from build123d import *

# Parameters (mm, degrees)
EXTRUDE_1_DEPTH     = 0.5
SKETCH_2_R          = 2
SKETCH_2_R_2        = 1.25
EXTRUDE_2_DEPTH     = 5.5
SKETCH_3_R          = 1.25
CUT_EXTRUDE_1_DEPTH = 5.5
SKETCH_4_R          = 4
SKETCH_4_R_2        = 2
CUT_EXTRUDE_2_DEPTH = 5.5


with BuildPart() as part:
    # 草图1 → 凸台-拉伸1 (new body)
    with BuildSketch(Plane.XY):
        with BuildLine():
            Line((0, 2), (3.2, 2))
            ThreePointArc((3.2, 2), (3.765685425, 2.234314575), (4, 2.8))
            Line((4, 2.8), (4, 2.95))
            ThreePointArc((4, 2.95), (3.765685425, 3.515685425), (3.2, 3.75))
            Line((3.2, 3.75), (-3.5, 3.75))
            Line((-3.5, 3.75), (-7, 2))
            Line((-7, 2), (-12.5, 2))
            Line((-12.5, 2), (-12.5, -2))
            Line((-12.5, -2), (-7, -2))
            Line((-7, -2), (-3.5, -3.75))
            Line((-3.5, -3.75), (3.2, -3.75))
            ThreePointArc((3.2, -3.75), (3.765685425, -3.515685425), (4, -2.95))
            Line((4, -2.95), (4, -2.8))
            ThreePointArc((4, -2.8), (3.765685425, -2.234314575), (3.2, -2))
            Line((3.2, -2), (0, -2))
            ThreePointArc((0, -2), (-2, 0), (0, 2))
        make_face()
    extrude(amount=EXTRUDE_1_DEPTH)

    # 草图2 → 凸台-拉伸2 (add)
    with BuildSketch(Plane.ZY.offset(12.5)):
        with Locations((1.5, 0)):
            Circle(SKETCH_2_R)
        with Locations((1.5, 0)):
            Circle(SKETCH_2_R_2, mode=Mode.SUBTRACT)
    extrude(amount=-EXTRUDE_2_DEPTH)

    # 草图3 → 切除-拉伸1 (cut)
    with BuildSketch(Plane.ZY.offset(12.5)):
        with Locations((1.5, 0)):
            Circle(SKETCH_3_R)
    extrude(amount=-CUT_EXTRUDE_1_DEPTH, mode=Mode.SUBTRACT)

    # 草图4 → 切除-拉伸2 (cut)
    with BuildSketch(Plane.ZY.offset(12.5)):
        with Locations((1.5, 0)):
            Circle(SKETCH_4_R)
        with Locations((1.5, 0)):
            Circle(SKETCH_4_R_2, mode=Mode.SUBTRACT)
    extrude(amount=-CUT_EXTRUDE_2_DEPTH, mode=Mode.SUBTRACT)


solid = part.part
Here's how the part is built. I have some questions about the finished solid (model axes, mm). A direction names the side the tool comes from. Round coordinates to 2 decimals unless told otherwise and drop trailing zeros. Write each loop counter-clockwise with the first axis right and the second up, starting at its lowest first coordinate (ties: lowest second). Pieces come first, ordered by that corner, then holes.
1. For faces 5 (the cylindrical face through (-2, 0, 0.2)), 6 (the flat face through (-3, 0, 0)), which set-ups out of +Z, -Z, +X, -X, +Y, -Y let a thin tool reach every point of the face, with its end or its side?
2. I need wall thicknesses on L1, parallel to Y at x = -10, z = 1.5; L2, parallel to Z at x = -11.1, y = 0; L3, parallel to Y at x = 1.5, z = 0.05. Which ranges of each line are inside material? Lowest first, please.
3. Will these pins go through, and if not, where does the flat tip stop? pin 1 Ø3 at (x, y) = (-5, -2) entering from +Z; pin 2 Ø0.9 at (y, z) = (0.5, 2.5) entering from +X; pin 3 Ø1.5 at (x, y) = (-9, 1.5) entering from +Z.
4. Suppose I cut it at B-B (z = 1.5). List the corners of the cut face in (x, y) for me.
5. Suppose I cut it at C-C (x = -2.25). List the corners of the cut face in (y, z) for me.
6. If we mould it in two halves opening along Z, with no side actions, what happens to faces 1 (the cylindrical face through (-9.79, 0.41, 0.32)), 2 (the cylindrical face through (-9.788, 1.352, 0.026)), 3 (the flat face through (-7, 0, 3)), 4 (the flat face through (-3, 0, 0.5))? For each: released by +Z, released by -Z, zero draft, split by the parting line, or undercut.
7. Suppose I cut it at D-D (z = 2.3). List the corners of the cut face in (x, y) for me, and give its area (3 significant figures).
8. Suppose I cut it at A-A (y = 0). List the corners of the cut face in (x, z) for me, and give its area (4 significant figures).
Answer sheet:
1. face 5: +Z, -Z, +X
1. face 6: -Z, +X, +Y, -Y
2. L1: y = -2 to -1.25, 1.25 to 2
2. L2: z = -0.5 to 0.25, 2.75 to 3.5
2. L3: y = -3.75 to -2, 2 to 3.75
3. pin 1: stops at z = 0.5
3. pin 2: stops at x = -7
3. pin 3: stops at z = 3.35
4. outline: (-12.5, -2) - (-7, -2) - (-7, -1.25) - (-12.5, -1.25) - close; (-12.5, 1.25) - (-7, 1.25) - (-7, 2) - (-12.5, 2) - close
5. outline: (-3.75, 0) - (3.75, 0) - (3.75, 0.5) - (-3.75, 0.5) - close
6. face 1: undercut
6. face 2: split by the parting line
6. face 3: zero draft
6. face 4: released by +Z
7. outline: (-12.5, -1.83) - (-7, -1.83) - (-7, -0.96) - (-12.5, -0.96) - close; (-12.5, 0.96) - (-7, 0.96) - (-7, 1.83) - (-12.5, 1.83) - close
7. area: 9.60 mm2
8. outline: (-12.5, -0.5) - (-7, -0.5) - (-7, 0) - (-2, 0) - (-2, 0.5) - (-7, 0.5) - (-7, 0.25) - (-12.5, 0.25) - close; (-12.5, 2.75) - (-7, 2.75) - (-7, 3.5) - (-12.5, 3.5) - close
8. area: 10.75 mm2
